from build123d import *

# Parameters (mm, degrees)
F1_DEPTH = 12.7
F2_R     = 90.4875
F3_DEPTH = 12.7
F5_D     = 6.35


with BuildPart() as f1:
    # F0 (on Top) → F1 (new body)
    with BuildSketch(Plane.XY):
        with BuildLine():
            Line((101.6, 101.6), (-101.6, 101.6))
            ThreePointArc((-101.6, 101.6), (-110.580256, 97.880256), (-114.3, 88.9))
            Line((-114.3, 88.9), (-114.3, -88.9))
            ThreePointArc((-114.3, -88.9), (-110.580256, -97.880256), (-101.6, -101.6))
            Line((-101.6, -101.6), (101.6, -101.6))
            ThreePointArc((101.6, -101.6), (110.580256, -97.880256), (114.3, -88.9))
            Line((114.3, -88.9), (114.3, 88.9))
            ThreePointArc((114.3, 88.9), (110.580256, 97.880256), (101.6, 101.6))
        make_face()
    extrude(amount=F1_DEPTH)

    # F2 (on face) → F3 (cut)
    with BuildSketch(Plane.XY.offset(12.7)):
        Circle(F2_R)
    extrude(amount=-F3_DEPTH, mode=Mode.SUBTRACT)

    # F5 (through all)
    with Locations(Plane.XY.offset(12.7)):
        with Locations((-88.9, 76.2), (88.9, 76.2), (88.9, -76.2), (-88.9, -76.2)):
            Hole(F5_D / 2)


solid = f1.part
Source: CAD feature listing. Evaluate the final solid. Frame: model axes, mm. Round coordinates to 2 decimals unless told otherwise and drop trailing zeros. Loops run counter-clockwise (first coordinate to the right, second up) from the corner with the lowest first, then second, coordinate; pieces in that order, holes last. Notation, with made-up numbers: (11.25, -13) -> (54.25, -13) arc R15 ccw to (54.25, -5) -> close; hole circle Ø4 at (-31, 16.5). An arc over 180 degrees is marked (long way). Answer as a JSON object with one key per item and string values. Group by question number.
Q1. Section query C-C (x = -71). Output: boundary loops of the cut face in (y, z), plus the area to 3 significant figures.
Q2. Mould query, pull axis X, two halves, no side actions, for faces 1 (the cylindrical face through (-110.68, -97.78, 6.26)), 2 (the cylindrical face through (110.48, -97.98, 6.26)), 3 (the cylindrical face through (91.24, 78.346, 6.261)). Classes: pulls with the +X half, pulls with the -X half, needs draft (parallel to the pull), parting line crosses it, or undercut.
Q3. Section query D-D (y = -76.2). Output: boundary loops of the cut face in (x, z) (3 decimals).
Q4. Section query A-A (y = 0). Output: boundary loops of the cut face in (x, z).
Q5. Ray query, line 1 (X direction, y = -75.5, z = 0.75); line 2 (Y direction, x = 0, z = 9.75); line 3 (X direction, y = -78, z = 5.25). Return the intervals inside material, ascending. Write a range as from..to.
Q6. Section query B-B (z = 2). State how many separate pieces and enclosed holes the cut face has, plus the area to 3 significant figures.
Completed:
{
 "1": {"outline": "(-101.6, 0) -> (-56.1, 0) -> (-56.1, 12.7) -> (-101.6, 12.7) -> close; (56.1, 0) -> (101.6, 0) -> (101.6, 12.7) -> (56.1, 12.7) -> close", "area": "1,160 mm²"},
 "2": {"face 1": "pulls with the -X half", "face 2": "pulls with the +X half", "face 3": "undercut"},
 "3": {"outline": "(-114.3, 0) -> (-92.075, 0) -> (-92.075, 12.7) -> (-114.3, 12.7) -> close; (-85.725, 0) -> (-48.801, 0) -> (-48.801, 12.7) -> (-85.725, 12.7) -> close; (48.801, 0) -> (85.725, 0) -> (85.725, 12.7) -> (48.801, 12.7) -> close; (92.075, 0) -> (114.3, 0) -> (114.3, 12.7) -> (92.075, 12.7) -> close"},
 "4": {"outline": "(-114.3, 0) -> (-90.49, 0) -> (-90.49, 12.7) -> (-114.3, 12.7) -> close; (90.49, 0) -> (114.3, 0) -> (114.3, 12.7) -> (90.49, 12.7) -> close"},
 "5": {"line 1": "-114.3..-92, -85.8..-49.88, 49.88..85.8, 92..114.3", "line 2": "-101.6..-90.49, 90.49..101.6", "line 3": "-114.3..-91.52, -86.28..-45.87, 45.87..86.28, 91.52..114.3"},
 "6": {"separate pieces": "1", "enclosed holes": "5", "area": "20,500 mm²"}
}
